Autodesk Inventor part; units mm, degrees
ref_plane "YZ Plane" through (0, 0, 0) normal (1, 0, 0) x (0, 1, 0)
ref_plane "XZ Plane" through (0, 0, 0) normal (0, 1, 0) x (-1, 0, 0)
ref_plane "XY Plane" through (0, 0, 0) normal (0, 0, 1) x (1, 0, 0)
sketch "Sketch1" plane through (0, 0, 0) normal (0, 1, 0) x (-1, 0, 0)
  line L0 (25, -30) -> (-25, -30)
  line L1 (-25, -30) -> (-25, 30)
  line L2 (-25, 30) -> (25, 30)
  line L3 (25, 30) -> (25, -30)
  point P0 (0, 0)
  dimension "d0" = 50
  dimension "d1" = 60
  dimension "d8" = 30
  dimension "d9" = 25
extrude "Extrusion1" add sketch "Sketch1" along normal blind 15
sketch "Sketch2" plane through (0, 15, 0) normal (0, 1, 0) x (1, 0, 0)
  line L0 (-16.85, 12.5) -> (16.85, 12.5)
  line L1 (16.85, 12.5) -> (16.85, -12.5)
  line L2 (16.85, -12.5) -> (-16.85, -12.5)
  line L3 (-16.85, -12.5) -> (-16.85, 12.5)
  point P0 (0, 0)
  dimension "d4" = 33.7
  dimension "d5" = 25
  dimension "d6" = 12.5
  dimension "d7" = 16.85
extrude "Extrusion2" cut sketch "Sketch2" against normal blind 10
sketch "Sketch3" plane through (0, 15, 0) normal (0, 1, 0) x (1, 0, 0)
  line L0 (-25, 30) -> (25, 30)
  line L1 (-25, -30) -> (25, -30)
  line L2 (-10, 30) -> (10, 30)
  line L3 (10, 30) -> (10, -30)
  line L4 (10, -30) -> (-10, -30)
  line L5 (-10, -30) -> (-10, 30)
  point P0 (0, 0)
  dimension "d12" = 20
  dimension "d13" = 10
extrude "Extrusion3" cut sketch "Sketch3" against normal up to surface (10 mm away)
sketch "Sketch4" plane through (0, 5, 0) normal (0, 1, 0) x (1, 0, 0)
  line L0 (-16.85, 12.5) -> (-10, 12.5)
  line L1 (16.85, -12.5) -> (10, -12.5)
  line L2 (10, 12.5) -> (10, 30)
  line L3 (-10, -30) -> (-10, -12.5)
  line L4 (10, 23) -> (-10, 23)
  line L5 (-10, 23) -> (-10, -23)
  line L6 (-10, -23) -> (10, -23)
  line L7 (10, -23) -> (10, 23)
  line L8 (-10, 30) -> (10, 30)
  line L9 (10, -30) -> (-10, -30)
  dimension "d18" = 7
  dimension "d19" = 7
extrude "Extrusion4" cut sketch "Sketch4" against normal up to next
sketch "Sketch6" plane through (-25, 0, -30) normal (-1, 0, 0) x (0, 0, 1)
  line L0 (0, 0) -> (0, 15)
  line L1 (60, 0) -> (60, 15)
  line L2 (60, 0) -> (0, 0)
  point P0 (30, 0)
  point P1 (10, 4)
  point P2 (50, 4)
  point P3 (50, 11)
  point P4 (10, 11)
  dimension "d24" = 7
  dimension "d25" = 7
  dimension "d26" = 10
  dimension "d27" = 10
  dimension "d28" = 10
  dimension "d29" = 10
  dimension "d30" = 4
  dimension "d31" = 4
hole "Hole1" at (-25, 4, -20) at (-25, 4, 20) at (-25, 11, 20) at (-25, 11, -20) direction (1, 0, 0) diameter 2.459 depth 7 tip angle 118
sketch "Sketch7" plane through (25, 0, 30) normal (1, 0, 0) x (0, 0, -1)
  circle A0 centre (10, 4) radius 1.2295
  circle A1 centre (10, 11) radius 1.2295
  circle A2 centre (50, 11) radius 1.2295
  circle A3 centre (50, 4) radius 1.2295
  point P0 (30, 0)
hole "Hole2" at (25, 4, 20) at (25, 11, 20) at (25, 11, -20) at (25, 4, -20) direction (-1, 0, 0) diameter 2.459 depth 7 tip angle 118
sketch "Sketch8" plane through (-25, 0, 30) normal (0, 0, 1) x (1, 0, 0)
  line L0 (0, 15) -> (15, 15)
  line L1 (8.15, 15) -> (41.85, 15)
  line L2 (41.85, 15) -> (41.85, 10)
  line L3 (41.85, 10) -> (8.15, 10)
  line L4 (8.15, 10) -> (8.15, 15)
  line L5 (41.85, 15) -> (41.85, 5)
  line L6 (8.15, 15) -> (8.15, 5)
  point P0 (25, 0)
  dimension "d49" = 5
  dimension "d50" = 0
  dimension "d51" = 0
  dimension "d52" = 0
extrude "Extrusion6" cut sketch "Sketch8" against normal through all
properties part number "Spring support"
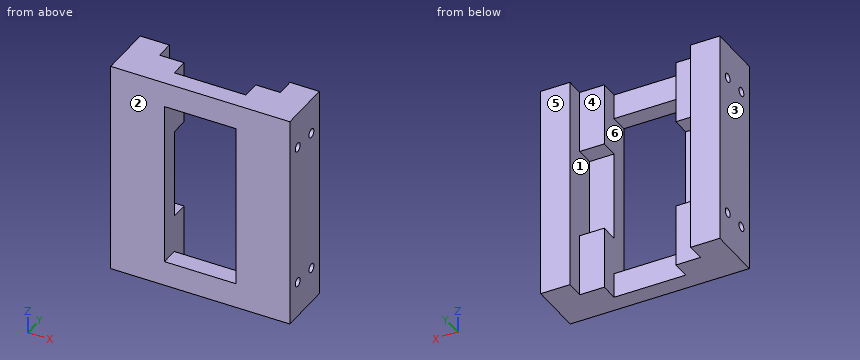
Can you work these out from the model? Positions are in its coordinate system, mm. Face numbers are marked on the shaded views. A direction names the side the tool comes from. Round coordinates to 2 decimals unless told otherwise and drop trailing zeros. Loops run counter-clockwise (first coordinate to the right, second up) from the corner with the lowest first, then second, coordinate; pieces in that order, holes last. Notation, with made-up numbers: M 13.5,20.25 L 43.5,20.25 A36 cw 43.5,55.25 Z; hole C 82.25,89 d6. An arc over 180 degrees is marked long. Write item = value, one per line. Start each with the question number.
(1) Which directions (+Z, -Z, +X, -X, +Y, -Y) give clear straight access to the entire face, cutting with the end or side of a thin tool? Please do the marked faces 4, 5 and 6.
(2) I need wall thicknesses on line 1 along Y through (x, z) = (-20, -20); line 2 along Z through (x, y) = (20.25, 11); line 3 along X through (y, z) = (8.5, -27). Which ranges of each line are inside material? Lowest first, please.
(3) Suppose I cut it at B-B on x = 19. Write out the boundary of the cut face in (y, z).
(4) Suppose I cut it at A-A on x = -0.5. Write out the boundary of the cut face in (y, z), plus the area to 3 significant figures.
(5) If we mould it in two halves opening along X, with no side actions, what happens to the marked faces 1, 2 and 3? For each: released by +X, released by -X, zero draft, split by the parting line, or undercut.
(6) Suppose I cut it at D-D on x = 12. Write out the boundary of the cut face in (y, z), plus the area to 3 significant figures.
(7) I'm going to push flat-ended pins straight in: P1, Ø2, axis at x = 0, z = 27.5, coming from the +Y side; P2, Ø2, axis at x = -15, z = 23.5, coming from the +Y side. Where does each tip first touch, or does it pass through?
(8) Suppose I cut it at C-C on z = 8.5. Write out the boundary of the cut face in (x, y).
Answer block:
q1.face_4 = +Z, -Z, +Y
q1.face_5 = +Z, -Z, +X, -X, +Y
q1.face_6 = +Y
q2.line_1 = 0 to 2.77, 5.23 to 9.77, 12.23 to 15
q2.line_2 = -30 to -21.23, -18.77 to 18.77, 21.23 to 30
q2.line_3 = -25 to -10, 10 to 25
q3.outline = M 0,-30 L 15,-30 L 15,30 L 0,30 Z; hole C 4,-20 d2.46; hole C 4,20 d2.46; hole C 11,-20 d2.46; hole C 11,20 d2.46
q4.outline = M 0,-30 L 5,-30 L 5,-23 L 0,-23 Z; M 0,23 L 5,23 L 5,30 L 0,30 Z
q4.area = 70.0 mm²
q5.face_1 = undercut
q5.face_2 = zero draft
q5.face_3 = released by -X
q6.outline = M 0,-30 L 10,-30 L 10,-12.5 L 5,-12.5 L 5,12.5 L 10,12.5 L 10,30 L 0,30 Z
q6.area = 475 mm²
q7.P1 = 5
q7.P2 = 10
q8.outline = M -25,0 L -10,0 L -10,5 L -16.85,5 L -16.85,15 L -25,15 Z; M 10,0 L 25,0 L 25,15 L 16.85,15 L 16.85,5 L 10,5 Z
